```python
from build123d import *

# Parameters (mm, degrees)
SKETCH1_W           = 146.03
SKETCH1_H           = 169.14
BOSS_EXTRUDE2_DEPTH = 52
SKETCH6_W           = 141.03
SKETCH6_H           = 164.14
CUT_EXTRUDE3_DEPTH  = 49
SKETCH7_R           = 2.16
CUT_EXTRUDE4_DEPTH  = 50
SKETCH8_R           = 4.5
CUT_EXTRUDE5_DEPTH  = 2.5
SKETCH9_W           = 16
SKETCH9_H           = 8
CUT_EXTRUDE6_DEPTH  = 3
SKETCH12_W          = 164.14
SKETCH12_H          = 49.5
CUT_EXTRUDE9_DEPTH  = 3
SKETCH13_R          = 3.95
CUT_EXTRUDE10_DEPTH = 3
SKETCH14_R          = 3
CUT_EXTRUDE11_DEPTH = 3


with BuildPart() as part:
    # Sketch1 → Boss-Extrude2 (new body)
    with BuildSketch(Plane(origin=(0, 0, 0), x_dir=(1, 0, 0), z_dir=(0, 1, 0))):
        with Locations((-17.115088028, 11.447931338)):
            Rectangle(SKETCH1_W, SKETCH1_H)
    extrude(amount=BOSS_EXTRUDE2_DEPTH)

    # Sketch6 → Cut-Extrude3 (cut)
    with BuildSketch(Plane(origin=(0, 52, 0), x_dir=(1, 0, 0), z_dir=(0, 1, 0))):
        with Locations((-17.115088028, 11.447931338)):
            Rectangle(SKETCH6_W, SKETCH6_H)
    extrude(amount=-CUT_EXTRUDE3_DEPTH, mode=Mode.SUBTRACT)

    # Sketch7 → Cut-Extrude4 (cut)
    with BuildSketch(Plane(origin=(0, 3, 0), x_dir=(1, 0, 0), z_dir=(0, 1, 0))):
        with Locations(Location((39.239911972, -56.462068662, 0), (0, 0, 270))):
            Circle(SKETCH7_R)
        with Locations(Location((39.239911972, 79.357931338, 0), (0, 0, 270))):
            Circle(SKETCH7_R)
        with Locations(Location((-29.370088028, 19.517931338, 0), (0, 0, 270))):
            Circle(SKETCH7_R)
    extrude(amount=-CUT_EXTRUDE4_DEPTH, mode=Mode.SUBTRACT)

    # Sketch8 → Cut-Extrude5 (cut)
    with BuildSketch(Plane(origin=(55.899911972, 0, 0), x_dir=(0, 0, -1), z_dir=(1, 0, 0))):
        with Locations((61.017931338, 39)):
            Circle(SKETCH8_R)
    extrude(amount=-CUT_EXTRUDE5_DEPTH, mode=Mode.SUBTRACT)

    # Sketch9 → Cut-Extrude6 (cut)
    with BuildSketch(Plane.XY.offset(73.122068662)):
        with Locations((25.899911972, 34)):
            Rectangle(SKETCH9_W, SKETCH9_H)
    extrude(amount=-CUT_EXTRUDE6_DEPTH, mode=Mode.SUBTRACT)

    # Sketch12 → Cut-Extrude9 (cut)
    with BuildSketch(Plane.ZY.offset(90.130088028)):
        with Locations((-11.447931338, 27.25)):
            Rectangle(SKETCH12_W, SKETCH12_H)
    extrude(amount=-CUT_EXTRUDE9_DEPTH, mode=Mode.SUBTRACT)

    # Sketch13 → Cut-Extrude10 (cut)
    with BuildSketch(Plane.XY.offset(73.122068662)):
        with Locations((-66.33891095, 42.5)):
            Circle(SKETCH13_R)
    extrude(amount=-CUT_EXTRUDE10_DEPTH, mode=Mode.SUBTRACT)

    # Sketch14 → Cut-Extrude11 (cut)
    with BuildSketch(Plane(origin=(0, 0, -96.017931338), x_dir=(-1, 0, 0), z_dir=(0, 0, -1))):
        with Locations((42.130088028, 24)):
            Circle(SKETCH14_R)
    extrude(amount=-CUT_EXTRUDE11_DEPTH, mode=Mode.SUBTRACT)


solid = part.part
```
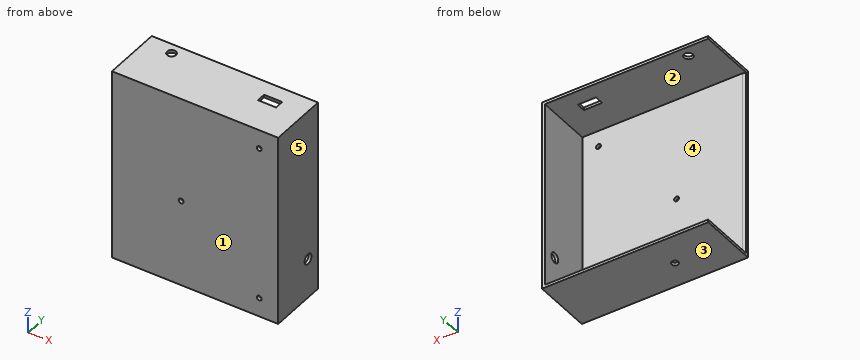
Geometry: final body of the model. Coordinates: model frame, mm. Face numbers are marked on the shaded views. A direction names the side the tool comes from. Give positions to 0.01 mm unless a question says otherwise; leave off trailing zeros. Write each loop counter-clockwise with the first axis right and the second up, starting at its lowest first coordinate (ties: lowest second). Pieces come first, ordered by that corner, then holes.
1. Pin query (flat end, axial travel): P1, Ø1.5, axis at y = 38, z = -21.5, coming from the -X side; P2, Ø7, axis at x = -29.37, z = -19.52, coming from the +Y side; P3, Ø1.5, axis at x = -89, z = 3.5, coming from the +Y side. Return the tip coordinate at first contact, or that it passes through.
2. Section query A-A, the plane y = 24. Return loops of the section in (x, z).
3. Section query C-C, the plane z = -13. Return loops of the section in (x, y).
4. Reachability of the marked faces 4 and 5 from +Z, -Z, +X, -X, +Y, -Y: full face, straight path, thin tool, end or side. Return the list, or none.
5. Section query B-B, the plane x = -52. Return loops of the section in (y, z).
6. Draft query along Z for the marked faces 1, 2 and 3. Return one class per face: released by +Z, released by -Z, zero draft, split by the parting line, or undercut.
7. Line query: probe 1 along Z at (x, y) = (-9, 42.5); probe 2 along Y at (x, z) = (-16, -36); probe 3 along X at (y, z) = (6, -48). Output: solid intervals per line, ascending.
Computed:
1. P1: stops at x = 53.4
1. P2: stops at y = 3
1. P3: stops at y = 2.5
2. outline: (-90.13, -96.02) - (-45.13, -96.02) - (-45.13, -93.52) - (-90.13, -93.52) - close; (-90.13, 70.62) - (53.4, 70.62) - (53.4, -93.52) - (-39.13, -93.52) - (-39.13, -96.02) - (55.9, -96.02) - (55.9, 73.12) - (-90.13, 73.12) - close
3. outline: (-90.13, 0) - (55.9, 0) - (55.9, 52) - (53.4, 52) - (53.4, 3) - (-87.13, 3) - (-87.13, 2.5) - (-90.13, 2.5) - close
4. face 4: -X, +Y
4. face 5: +Z, -Z, +X, +Y, -Y
5. outline: (0, -96.02) - (52, -96.02) - (52, -93.52) - (3, -93.52) - (3, 70.62) - (52, 70.62) - (52, 73.12) - (0, 73.12) - close
6. face 1: zero draft
6. face 2: undercut
6. face 3: released by -Z
7. probe 1: z = -96.02 to -93.52, 70.62 to 73.12
7. probe 2: y = 0 to 3
7. probe 3: x = 53.4 to 55.9
